from build123d import *

# Parameters (mm, degrees)
BOSS_EXTRUDE1_DEPTH     = 280
BOSS_EXTRUDE3_START     = 10
BOSS_EXTRUDE3_DEPTH     = 10
CUT_EXTRUDE_THIN1_START = -2
CUT_EXTRUDE_THIN1_DEPTH = 2
FILLET6_R               = 1


# Read off the part's stored shape, not the designer's step: Cut-Extrude-Thin1
with BuildPart() as part:
    # Sketch1 → Boss-Extrude1 (new body)
    with BuildSketch(Plane.XY):
        with BuildLine():
            Line((0, 55), (-2, 55))
            Line((-2, 55), (-2, 51.5))
            Line((-2, 51.5), (0, 51.5))
            Line((0, 51.5), (0, 50.5))
            ThreePointArc((0, 50.5), (-50.5, 0), (0, -50.5))
            Line((0, -50.5), (0, -51.5))
            Line((0, -51.5), (-2, -51.5))
            Line((-2, -51.5), (-2, -55))
            Line((-2, -55), (0, -55))
            Line((0, -55), (0, -60))
            ThreePointArc((0, -60), (-60, 0), (0, 60))
            Line((0, 60), (0, 55))
        make_face()
    extrude(amount=-BOSS_EXTRUDE1_DEPTH)

    # Sketch7 → Boss-Extrude3 (add)
    with BuildSketch(Plane.XY.offset(BOSS_EXTRUDE3_START)):
        with BuildLine():
            Line((0, 60), (0, -60))
            ThreePointArc((0, -60), (-60, 0), (0, 60))
        make_face()
    boss_extrude3 = extrude(amount=-BOSS_EXTRUDE3_DEPTH)

    # Mirror1: Boss-Extrude3 across plane
    add(boss_extrude3.mirror(Plane.XY.offset(-140)))

    # Cut-Extrude-Thin1 outline → Cut-Extrude-Thin1 (cut)
    with BuildSketch(Plane(origin=(0, 0, 0), x_dir=(0, 0, -1), z_dir=(1, 0, 0)).offset(CUT_EXTRUDE_THIN1_START)):
        Polygon((0, 55), (-7, 55), (-7, -55), (0, -55), (0, -51.5), (-3.5, -51.5), (-3.5, 51.5), (0, 51.5), align=None)
    cut_extrude_thin1 = extrude(amount=CUT_EXTRUDE_THIN1_DEPTH, mode=Mode.SUBTRACT)

    # Mirror2: Cut-Extrude-Thin1 across plane
    add(cut_extrude_thin1.mirror(Plane.XY.offset(-140)), mode=Mode.SUBTRACT)

    # Fillet6
    fillet6_edges = [part.edges().sort_by_distance(p)[0] for p in [
        (-1, -55, 7),
        (-1, 55, 7),
        (-1, 51.5, 3.5),
        (-1, -51.5, 3.5),
        (-1, -55, -287),
        (-1, -51.5, -283.5),
        (-1, 51.5, -283.5),
        (-1, 55, -287),
    ]]
    fillet(fillet6_edges, radius=FILLET6_R)


solid = part.part
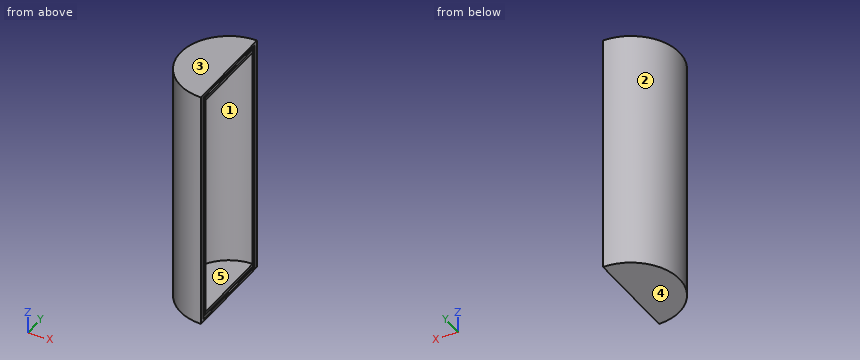
Work out the finished part from the listing and answer in its coordinate system (mm). Face numbers are marked on the shaded views. A direction names the side the tool comes from. Coordinates: 2 decimals unless noted, no trailing zeros. Write each loop counter-clockwise with the first axis right and the second up, starting at its lowest first coordinate (ties: lowest second). Pieces come first, ordered by that corner, then holes. Notation, with made-up numbers: M -24,-13.5 L 16,-13.5 A32 ccw 16,18.5 Z; hole C 35.5,34 d3. An arc over 180 degrees is marked long. Use one line per item in the form item = value. Start each with the question number.
1. Each of these flat-tipped pins is pushed along its axis until it touches: P1, Ø2, axis at y = 33, z = -119, coming from the +X side; P2, Ø4, axis at y = -25, z = -126.5, coming from the -X side; P3, Ø2, axis at y = 22, z = -95, coming from the -X side (3 decimals). Where does it stop, or does it pass through?
2. The mould has two halves that part along Z. Classify the marked faces 1, 2 and 3: released by +Z, released by -Z, zero draft, split by the parting line, or undercut.
3. The part is cut by section B-B (z = -32). Give the vertices of the cut face in (x, y).
4. The part is cut by section C-C (x = -25.5). Give the vertices of the cut face in (y, z), plus the area to 3 significant figures.
5. The part is cut by section A-A (y = 0). Give the vertices of the cut face in (x, z), plus the area to 3 significant figures.
6. The part is cut by section D-D (y = -46.5). Give the vertices of the cut face in (x, z), plus the area to 3 significant figures.
7. A tool of negligible diameter and unlimited length cuts with its end or side. For the marked faces 4 and 5, from which of +Z, -Z, +X, -X, +Y, -Y can it reach the whole face along a straight path? Write none if from no direction.
8. Straight lines are drawn through the part: probe 1 along Z at (x, y) = (-12, 43); probe 2 along Y at (x, z) = (-31.5, -9); probe 3 along Y at (x, z) = (-42, -4). For each, find the intervals that lie inside material, in ascending order. Write a range as from..to.
Evaluation:
q1.P1 = -37.34
q1.P2 = -55.42
q1.P3 = -56.205
q2.face_1 = undercut
q2.face_2 = zero draft
q2.face_3 = released by +Z
q3.outline = M -2,-55 L -2,-51.5 L 0,-51.5 L 0,-50.5 A50.5 cw 0,50.5 L 0,51.5 L -2,51.5 L -2,55 L 0,55 L 0,60 A60 ccw 0,-60 L 0,-55 Z
q4.outline = M -54.31,-290 L 54.31,-290 L 54.31,10 L -54.31,10 Z; hole M -43.59,-280 L 43.59,-280 L 43.59,0 L -43.59,0 Z
q4.area = 8,180 mm^2
q5.outline = M -60,-290 L 0,-290 L 0,-287 L -2,-287 L -2,-283.5 L 0,-283.5 L 0,-280 L -50.5,-280 L -50.5,0 L 0,0 L 0,3.5 L -2,3.5 L -2,7 L 0,7 L 0,10 L -60,10 Z
q5.area = 3,850 mm^2
q6.outline = M -37.92,-290 L 0,-290 L 0,-287 L -2,-287 L -2,-283.5 L 0,-283.5 L 0,-280 L -19.7,-280 L -19.7,0 L 0,0 L 0,3.5 L -2,3.5 L -2,7 L 0,7 L 0,10 L -37.92,10 Z
q6.area = 5,850 mm^2
q7.face_4 = -Z, +X, -X, +Y, -Y
q7.face_5 = +X
q8.probe_1 = -290..-280, 0..10
q8.probe_2 = -51.07..-39.47, 39.47..51.07
q8.probe_3 = -42.85..-28.04, 28.04..42.85
